For this review, take the finished solid that the model builds, in its own axes (mm). A direction names the side the tool comes from. Coordinates: 2 decimals unless noted, no trailing zeros. Write each loop counter-clockwise with the first axis right and the second up, starting at its lowest first coordinate (ties: lowest second). Pieces come first, ordered by that corner, then holes.
1) To check wall thickness, follow line 1 along Y through (x, z) = (96, -16); line 2 along Z through (x, y) = (19.5, 6.5); line 3 along X through (y, z) = (12, -17). State the ranges of each line that lie inside material, in increasing order.
2) We need section C-C on x = -78.5. Write out the cut boundary in (y, z) (3 decimals).
3) We need section A-A on z = 9.5. Write out the cut boundary in (x, y).
4) Mouldability with a two-part tool opening along Z and no side actions: class faces 1 (the face through (3, 0, 19.05)), 2 (the face through (12, 16.51, 0)), 3 (the face through (3, 0, -16.51)), 4 (the face through (-103.455, -0.267, -16.667)) as pulls with the +Z half, pulls with the -Z half, needs draft (parallel to the pull), parting line crosses it, or undercut.
5) For faces 5 (the face through (3, 0, 16.51)), 6 (the face through (2, -19.05, 0)), list the 3-axis set-ups (+Z, -Z, +X, -X, +Y, -Y) from which the entire face can be reached by the end or side of a thin tool; tool diameter is ignored.
6) We need section B-B on y = 7. Write out the cut boundary in (x, z), then the cut area to 3 significant figures.
from build123d import *

# Parameters (mm, degrees)
EXTRUDE_THIN1_DEPTH     = 114.3
CUT_EXTRUDE1_DEPTH      = 1
CUT_EXTRUDE1_DEPTH_BACK = 39.1


with BuildPart() as part:
    # Sketch1 → Extrude-Thin1 (new body, symmetric)
    with BuildSketch(Plane(origin=(0, 0, 0), x_dir=(0, 0, -1), z_dir=(1, 0, 0))):
        with BuildLine():
            Line((-15.875, 19.05), (15.875, 19.05))
            ThreePointArc((15.875, 19.05), (18.12006403, 18.12006403), (19.05, 15.875))
            Line((19.05, 15.875), (19.05, -15.875))
            ThreePointArc((19.05, -15.875), (18.12006403, -18.12006403), (15.875, -19.05))
            Line((15.875, -19.05), (-15.875, -19.05))
            ThreePointArc((-15.875, -19.05), (-18.12006403, -18.12006403), (-19.05, -15.875))
            Line((-19.05, -15.875), (-19.05, 15.875))
            ThreePointArc((-19.05, 15.875), (-18.12006403, 18.12006403), (-15.875, 19.05))
        make_face()
        with BuildLine():
            Line((-15.875, 16.51), (15.875, 16.51))
            ThreePointArc((15.875, 16.51), (16.324012806, 16.324012806), (16.51, 15.875))
            Line((16.51, 15.875), (16.51, -15.875))
            ThreePointArc((16.51, -15.875), (16.324012806, -16.324012806), (15.875, -16.51))
            Line((15.875, -16.51), (-15.875, -16.51))
            ThreePointArc((-15.875, -16.51), (-16.324012806, -16.324012806), (-16.51, -15.875))
            Line((-16.51, -15.875), (-16.51, 15.875))
            ThreePointArc((-16.51, 15.875), (-16.324012806, 16.324012806), (-15.875, 16.51))
        make_face(mode=Mode.SUBTRACT)
    extrude(amount=EXTRUDE_THIN1_DEPTH, both=True)

    # Sketch2 → Cut-Extrude1 (cut, two sides)
    with BuildSketch(Plane.XY.offset(19.05)) as cut_extrude1_sk:
        Polygon((-351.053252404, -429.118662022), (-114.3, -19.05), (-92.302954744, 19.05), (144.45029766, 429.118662022), (-675.687026383, 902.62516683), (-1171.190576447, 44.387842787), align=None)
    extrude(amount=CUT_EXTRUDE1_DEPTH, mode=Mode.SUBTRACT)
    extrude(cut_extrude1_sk.sketch, amount=-CUT_EXTRUDE1_DEPTH_BACK, mode=Mode.SUBTRACT)


solid = part.part
Result:
1. line 1: y = -19.05 to -16.5, 16.5 to 19.05
1. line 2: z = -19.05 to -16.51, 16.51 to 19.05
1. line 3: x = -96.37 to 114.3
2. outline: (-19.05, -15.875) arc R3.175 ccw to (-15.875, -19.05) - (15.875, -19.05) arc R3.175 ccw to (19.05, -15.875) - (19.05, 15.875) arc R3.175 ccw to (15.875, 19.05) - (-15.875, 19.05) arc R3.175 ccw to (-19.05, 15.875) - close; hole (-16.51, -15.875) arc R0.635 ccw to (-15.875, -16.51) - (15.875, -16.51) arc R0.635 ccw to (16.51, -15.875) - (16.51, 15.875) arc R0.635 ccw to (15.875, 16.51) - (-15.875, 16.51) arc R0.635 ccw to (-16.51, 15.875) - close
3. outline: (-114.3, -19.05) - (114.3, -19.05) - (114.3, -16.51) - (-112.83, -16.51) - close; (-93.77, 16.51) - (114.3, 16.51) - (114.3, 19.05) - (-92.3, 19.05) - close
4. face 1: pulls with the +Z half
4. face 2: undercut
4. face 3: undercut
4. face 4: needs draft
5. face 5: +X, -X
5. face 6: +Z, -Z, +X, -X, -Y
6. outline: (-99.26, -19.05) - (114.3, -19.05) - (114.3, -16.51) - (-99.26, -16.51) - close; (-99.26, 16.51) - (114.3, 16.51) - (114.3, 19.05) - (-99.26, 19.05) - close
6. area: 1,080 mm2
